The listing builds one solid part. Answer for the finished solid, in the listing's coordinates (mm). A direction names the side the tool comes from. Round coordinates to 2 decimals unless told otherwise and drop trailing zeros. Loops run counter-clockwise (first coordinate to the right, second up) from the corner with the lowest first, then second, coordinate; pieces in that order, holes last. Notation, with made-up numbers: (52.25, 77) -> (70.25, 77) arc R20 cw to (70.25, 89) -> close; hole circle Ø8 at (-10, 25.5). An arc over 180 degrees is marked (long way). Write each question's results on one line, items separated by ' | '. Start each with the question number.
from build123d import *

# Parameters (mm, degrees)
ODGI_CIE_BAZOWE1_DEPTH     = 50
SZKIC6_W                   = 26
SZKIC6_H                   = 47
WYTNIJ_WYCI_GNI_CIE1_DEPTH = 94.541434669
OTW_R_POD_RUB_M51_D        = 5.5
OTW_R_POD_RUB_M52_D        = 5.5
SZKIC11_W                  = 17
SZKIC11_H                  = 18
WYTNIJ_WYCI_GNI_CIE2_DEPTH = 93.135769384
SFAZOWANIE1_SIZE           = 5
SFAZOWANIE1_SIZE2          = 8.660254038
ZAOKR_GLENIE1_R            = 4


# Sheet-metal steps are written as plain solids
with BuildPart() as part:
    # Szkic1 → Odgięcie bazowe1 (new, symmetric)
    with BuildSketch(Plane(origin=(0, 0, 0), x_dir=(0, 0, -1), z_dir=(1, 0, 0))):
        with BuildLine():
            Line((-65, 0), (-7, 0))
            ThreePointArc((-7, 0), (-2.050252532, 2.050252532), (0, 7))
            Line((0, 7), (0, 45))
            Line((0, 45), (-3, 45))
            Line((-3, 45), (-3, 7))
            ThreePointArc((-3, 7), (-4.171572875, 4.171572875), (-7, 3))
            Line((-7, 3), (-65, 3))
            Line((-65, 3), (-65, 0))
        make_face()
    extrude(amount=ODGI_CIE_BAZOWE1_DEPTH, both=True)

    # Szkic6 → Wytnij-wyciągnięcie1 (cut, through all)
    with BuildSketch(Plane.XZ):
        with Locations((37, 23.5)):
            Rectangle(SZKIC6_W, SZKIC6_H)
        with Locations((-37, 23.5)):
            Rectangle(SZKIC6_W, SZKIC6_H)
    extrude(amount=-WYTNIJ_WYCI_GNI_CIE1_DEPTH, mode=Mode.SUBTRACT)

    # Otwór pod śrubę M51 (through all)
    with Locations(Plane(origin=(0, 0, 0), x_dir=(-1, 0, 0), z_dir=(0, 0, -1))):
        with Locations((0, 30), (-12.5, 20), (12.5, 20)):
            Hole(OTW_R_POD_RUB_M51_D / 2)

    # Otwór pod śrubę M52 (through all)
    with Locations(Plane(origin=(0, 0, 0), x_dir=(-1, 0, 0), z_dir=(0, -1, 0))):
        with Locations((20, -55), (-20, -55)):
            Hole(OTW_R_POD_RUB_M52_D / 2)

    # Szkic11 → Wytnij-wyciągnięcie2 (cut, through all)
    with BuildSketch(Plane(origin=(0, 3, 0), x_dir=(1, 0, 0), z_dir=(0, 1, 0))):
        with Locations((-41.5, -56)):
            Rectangle(SZKIC11_W, SZKIC11_H)
    extrude(amount=-WYTNIJ_WYCI_GNI_CIE2_DEPTH, mode=Mode.SUBTRACT)

    # Sfazowanie1
    sfazowanie1_edges = [part.edges().sort_by_distance(p)[0] for p in [
        (50, 1.5, 47),
    ]]
    sfazowanie1_side = [part.faces().sort_by_distance(p)[0] for p in [
        (50, 1.5, 56),
    ]]
    chamfer(sfazowanie1_edges, length=SFAZOWANIE1_SIZE, length2=SFAZOWANIE1_SIZE2, reference=sfazowanie1_side[0])

    # Zaokrąglenie1
    zaokr_glenie1_edges = [part.edges().sort_by_distance(p)[0] for p in [
        (-33, 1.5, 47),
        (-33, 1.5, 65),
        (-24, 45, 1.5),
        (-24, 1.5, 47),
        (24, 1.5, 47),
        (24, 45, 1.5),
        (50, 1.5, 65),
    ]]
    fillet(zaokr_glenie1_edges, radius=ZAOKR_GLENIE1_R)


solid = part.part
Item 1: For faces 1 (the flat face through (24, 2, 12)), 2 (the flat face through (0, 3, 42)), 3 (the cylindrical face through (-31.797, 1.479, 63.859)), determine the directions among +Z, -Z, +X, -X, +Y, -Y from which every point of the face is accessible in a straight line to the end or side of a thin tool.
Item 2: Determine the mould class of faces 4 (the cylindrical face through (19.642, 1.521, 52.273)), 5 (the cylindrical face through (0.336, 4.203, 4.141)), 6 (the cylindrical face through (22.859, 43.797, 1.479)) for opening direction Z: +Z half, -Z half, draft (parallel to the pull), parting line (faces both ways), or undercut.
Item 3: The part is cut by section A-A, the plane x = -12.5. Give the vertices of the cut face in (y, z).
Item 4: The part is cut by section D-D, the plane y = 20. Give the vertices of the cut face in (x, z).
Item 5: The part is cut by section C-C, the plane z = 55. Give the vertices of the cut face in (x, y).
Item 6: Each of these flat-tipped pins is pushed along its axis until it touches: pin 1 Ø5 at (x, y) = (-1.5, 10) entering from +Z; pin 2 Ø1.5 at (x, y) = (37, 1) entering from -Z; pin 3 Ø7 at (x, y) = (12.5, 20) entering from -Z; pin 4 Ø17.5 at (x, z) = (3.5, 37.5) entering from +Y. Where does it stop, or does it pass through?
Item 7: The part is cut by section B-B, the plane y = 30. Give the vertices of the cut face in (x, z), plus the area to 4 significant figures.
Item 8: Straight lines are drawn through the part: L1, parallel to Z at x = 20, y = 1.45; L2, parallel to Y at x = 18, z = 35. For each, find the intervals that lie inside material, in ascending order. Write a range as [from, to].
Report:
1) face 1: -Z, +X, +Y, -Y | face 2: +Z, +X, -X, +Y | face 3: +Z, -X, +Y, -Y
2) face 4: undercut | face 5: +Z half | face 6: draft
3) outline: (0, 7) arc R7 ccw to (7, 0) -> (17.25, 0) -> (17.25, 3) -> (7, 3) arc R4 cw to (3, 7) -> (3, 65) -> (0, 65) -> close; (22.75, 0) -> (45, 0) -> (45, 3) -> (22.75, 3) -> close
4) outline: (-24, 0) -> (-15.25, 0) -> (-15.25, 3) -> (-24, 3) -> close; (-9.75, 0) -> (9.75, 0) -> (9.75, 3) -> (-9.75, 3) -> close; (15.25, 0) -> (24, 0) -> (24, 3) -> (15.25, 3) -> close
5) outline: (-33, 0) -> (-22.75, 0) -> (-22.75, 3) -> (-33, 3) -> close; (-17.25, 0) -> (17.25, 0) -> (17.25, 3) -> (-17.25, 3) -> close; (22.75, 0) -> (50, 0) -> (50, 3) -> (22.75, 3) -> close
6) pin 1: stops at z = 3 | pin 2: stops at z = 47 | pin 3: stops at z = 0 | pin 4: stops at y = 3
7) outline: (-24, 0) -> (-2.75, 0) -> (-2.75, 3) -> (-24, 3) -> close; (2.75, 0) -> (24, 0) -> (24, 3) -> (2.75, 3) -> close | area: 127.5 mm2
8) L1: z = [2.73, 52.25], [57.75, 65] | L2: y = [0, 3]
